Read the model definition and answer for the solid it produces. Units are mm, in the model's axes. Face numbers are marked on the shaded views. Coordinates: 2 decimals unless noted, no trailing zeros. Write each loop counter-clockwise with the first axis right and the second up, starting at its lowest first coordinate (ties: lowest second). Pieces come first, ordered by that corner, then holes.
Item 1: Straight lines are drawn through the part: probe 1 along Y at (x, z) = (2, 4.75); probe 2 along Y at (x, z) = (3, 6.75); probe 3 along Y at (x, z) = (4.5, 2.5). For each, find the intervals that lie inside material, in ascending order.
Item 2: Section D-D (y = 16.5) is taken. Give the vertices of the cut face in (x, z), then the cut area to 3 significant figures.
Item 3: Section C-C (y = 12.5) is taken. Give the vertices of the cut face in (x, z), then the cut area to 3 significant figures.
Item 4: Section A-A (x = 4.75) is taken. Give the vertices of the cut face in (y, z).
Item 5: This flat-tipped pin is pushed along its axis until it touches: P1, Ø3.5, axis at y = 5.5, z = 4.1, coming from the -X side. Where does it stop, or does it pass through?
Item 6: Section B-B (z = 4.1) is taken. Give the vertices of the cut face in (x, y).
Item 7: Determine the mould class of the marked faces 1, 2 and 3 for opening direction Z: released by +Z, released by -Z, zero draft, split by the parting line, or undercut.
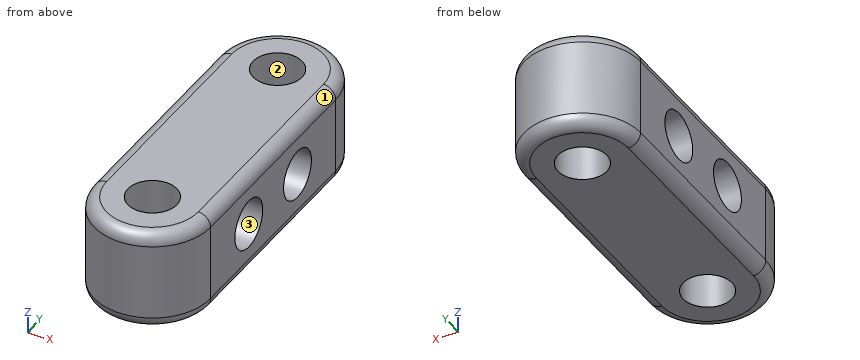
from build123d import *

# Parameters (mm, degrees)
BASE_EXTRUSION_DEPTH    = 8.2
ESQUISSE2_R             = 2
ENL_V_MAT_EXTRU_1_DEPTH = 26.981772457
CONG_1_R                = 1
CONG_2_R                = 1
ESQUISSE3_R             = 2
ENL_V_MAT_EXTRU_2_DEPTH = 26.981772457


with BuildPart() as part:
    # Esquisse1 → Base-Extrusion (new body)
    with BuildSketch(Plane.XY):
        with BuildLine():
            Line((0, 0), (0, 18))
            ThreePointArc((0, 18), (4.75, 22.75), (9.5, 18))
            Line((9.5, 18), (9.5, 0))
            ThreePointArc((9.5, 0), (4.75, -4.75), (0, 0))
        make_face()
    extrude(amount=BASE_EXTRUSION_DEPTH)

    # Esquisse2 → Enlèv. mat.-Extru.1 (cut, through all)
    with BuildSketch(Plane.XY.offset(8.2)):
        with Locations((4.75, 18)):
            Circle(ESQUISSE2_R)
        with Locations((4.75, 0)):
            Circle(ESQUISSE2_R)
    extrude(amount=-ENL_V_MAT_EXTRU_1_DEPTH, mode=Mode.SUBTRACT)

    # Congé1
    cong_1_edges = [part.edges().sort_by_distance(p)[0] for p in [
        (4.75, 22.75, 8.2),
        (0, 9, 8.2),
        (4.75, -4.75, 8.2),
        (9.5, 9, 8.2),
    ]]
    fillet(cong_1_edges, radius=CONG_1_R)

    # Congé2
    cong_2_edges = [part.edges().sort_by_distance(p)[0] for p in [
        (0, 9, 0),
        (4.75, 22.75, 0),
        (9.5, 9, 0),
        (4.75, -4.75, 0),
    ]]
    fillet(cong_2_edges, radius=CONG_2_R)

    # Esquisse3 → Enlèv. mat.-Extru.2 (cut, through all)
    with BuildSketch(Plane(origin=(9.5, 0, 0), x_dir=(0, 0, -1), z_dir=(1, 0, 0))):
        with Locations(Location((-4.1, 12.5, 0), (0, 0, 90))):
            Circle(ESQUISSE3_R)
        with Locations(Location((-4.1, 5.5, 0), (0, 0, 90))):
            Circle(ESQUISSE3_R)
    extrude(amount=-ENL_V_MAT_EXTRU_2_DEPTH, mode=Mode.SUBTRACT)


solid = part.part
Established:
1. probe 1: y = -3.87 to 3.61, 7.39 to 10.61, 14.39 to 21.87
1. probe 2: y = -4.42 to -0.97, 0.97 to 17.03, 18.97 to 22.42
1. probe 3: y = -4.74 to -1.98, 1.98 to 4.3, 6.7 to 11.3, 13.7 to 16.02, 19.98 to 22.74
2. outline: (0, 1) arc R1 ccw to (1, 0) - (3.43, 0) - (3.43, 8.2) - (1, 8.2) arc R1 ccw to (0, 7.2) - close; (6.07, 0) - (8.5, 0) arc R1 ccw to (9.5, 1) - (9.5, 7.2) arc R1 ccw to (8.5, 8.2) - (6.07, 8.2) - close
2. area: 55.3 mm2
3. outline: (0, 1) arc R1 ccw to (1, 0) - (8.5, 0) arc R1 ccw to (9.5, 1) - (9.5, 2.1) - (0, 2.1) - close; (0, 6.1) - (9.5, 6.1) - (9.5, 7.2) arc R1 ccw to (8.5, 8.2) - (1, 8.2) arc R1 ccw to (0, 7.2) - close
3. area: 39.0 mm2
4. outline: (-4.75, 1) arc R1 ccw to (-3.75, 0) - (-2, 0) - (-2, 8.2) - (-3.75, 8.2) arc R1 ccw to (-4.75, 7.2) - close; (2, 0) - (16, 0) - (16, 8.2) - (2, 8.2) - close; (20, 0) - (21.75, 0) arc R1 ccw to (22.75, 1) - (22.75, 7.2) arc R1 ccw to (21.75, 8.2) - (20, 8.2) - close; hole circle Ø4 at (5.5, 4.1); hole circle Ø4 at (12.5, 4.1)
5. P1: passes through
6. outline: (0, 0) arc R4.75 ccw to (9.5, 0) - (9.5, 3.5) - (0, 3.5) - close; (0, 7.5) - (9.5, 7.5) - (9.5, 10.5) - (0, 10.5) - close; (0, 14.5) - (9.5, 14.5) - (9.5, 18) arc R4.75 ccw to (0, 18) - close; hole circle Ø4 at (4.75, 0); hole circle Ø4 at (4.75, 18)
7. face 1: released by +Z
7. face 2: zero draft
7. face 3: undercut
